Geometry: final body of the model. Coordinates: model frame, mm. Face numbers are marked on the shaded views. A direction names the side the tool comes from. Round coordinates to 2 decimals unless told otherwise and drop trailing zeros. Loops run counter-clockwise (first coordinate to the right, second up) from the corner with the lowest first, then second, coordinate; pieces in that order, holes last. Notation, with made-up numbers: M 65,24 L 85,24 A22 cw 85,47 Z; hole C 7.25,55 d4. An arc over 180 degrees is marked long. Answer as a JSON object with one key per item and string values.
```python
from build123d import *

# Parameters (mm, degrees)
SKETCH1_W           = 60
SKETCH1_H           = 100
SKETCH1_W_2         = 150
SKETCH1_H_2         = 12
BOSS_EXTRUDE1_DEPTH = 30
FILLET1_R           = 10
SKETCH2_W           = 25
SKETCH2_H           = 10
SKETCH2_H_2         = 5
CUT_EXTRUDE1_DEPTH  = 222
FILLET2_R           = 5
SKETCH3_R           = 2
CUT_EXTRUDE2_DEPTH  = 51
SKETCH4_R           = 4
CUT_EXTRUDE3_DEPTH  = 4.5


with BuildPart() as part:
    # Sketch1 → Boss-Extrude1 (new body)
    with BuildSketch(Plane.XY):
        Rectangle(SKETCH1_W, SKETCH1_H)
        with Locations((0, -50)):
            Rectangle(SKETCH1_W_2, SKETCH1_H_2)
    extrude(amount=BOSS_EXTRUDE1_DEPTH)

    # Fillet1
    fillet1_edges = [part.edges().sort_by_distance(p)[0] for p in [
        (-30, -44, 15),
        (30, -44, 15),
    ]]
    fillet(fillet1_edges, radius=FILLET1_R)

    # Sketch2 → Cut-Extrude1 (cut)
    with BuildSketch(Plane(origin=(0, 50, 0), x_dir=(1, 0, 0), z_dir=(0, 1, 0))):
        with Locations((0, -5)):
            Rectangle(SKETCH2_W, SKETCH2_H)
        with Locations((0, -12.5)):
            Rectangle(SKETCH2_W, SKETCH2_H_2)
        Polygon((17.5, -10), (12.5, -10), (12.5, -15), (-12.5, -15), (-12.5, -10), (-17.5, -10), (-17.5, -20), (17.5, -20), align=None)
    extrude(amount=-CUT_EXTRUDE1_DEPTH, mode=Mode.SUBTRACT)

    # Fillet2
    fillet2_edges = [part.edges().sort_by_distance(p)[0] for p in [
        (12.5, 50, 5),
        (-12.5, 50, 5),
        (0, 50, 20),
        (-17.5, 50, 15),
        (17.5, 50, 15),
    ]]
    fillet(fillet2_edges, radius=FILLET2_R)

    # Sketch3 → Cut-Extrude2 (cut)
    with BuildSketch(Plane(origin=(0, -44, 0), x_dir=(1, 0, 0), z_dir=(0, 1, 0))):
        with Locations(Location((-57.5, -15, 0), (0, 0, 270))):
            Circle(SKETCH3_R)
    cut_extrude2 = extrude(amount=-CUT_EXTRUDE2_DEPTH, mode=Mode.SUBTRACT)

    # Sketch4 → Cut-Extrude3 (cut)
    with BuildSketch(Plane(origin=(0, -44, 0), x_dir=(1, 0, 0), z_dir=(0, 1, 0))):
        with Locations(Location((-57.5, -15, 0), (0, 0, 270))):
            Circle(SKETCH4_R)
    cut_extrude3 = extrude(amount=-CUT_EXTRUDE3_DEPTH, mode=Mode.SUBTRACT)

    # Mirror1: Cut-Extrude2, Cut-Extrude3 across plane
    add(cut_extrude2.mirror(Plane(origin=(0, 0, 0), x_dir=(0, 0, 1), z_dir=(1, 0, 0))), mode=Mode.SUBTRACT)
    add(cut_extrude3.mirror(Plane(origin=(0, 0, 0), x_dir=(0, 0, 1), z_dir=(1, 0, 0))), mode=Mode.SUBTRACT)


solid = part.part
```
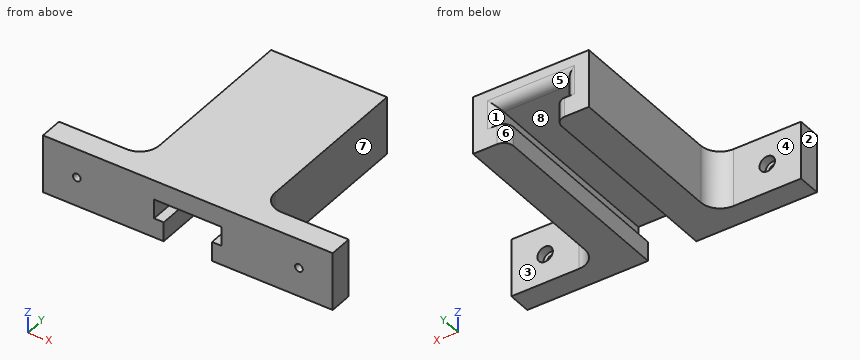
1) First-contact query: pin 1 (9 mm diameter, centred on x = 55.5, z = 15.5, fed in from +Y); pin 2 (11 mm diameter, centred on y = -30, z = 13, fed in from -X); pin 3 (9 mm diameter, centred on x = -57.5, z = 15, fed in from -Y); pin 4 (1 mm diameter, centred on y = 37.5, z = 4, fed in from +X). Flat tips, straight axial feed; report the tip coordinate or a pass-through.
Geometry results:
{"pin 1": "y = -44", "pin 2": "x = -30.11", "pin 3": "y = -56", "pin 4": "x = 30"}
2) Pull-direction query (X, two-part tool) for the marked faces 1, 2 and 3; classes: +X half, -X half, draft (parallel to the pull), parting line (faces both ways), or undercut.
Geometry results:
{"face 1": "undercut", "face 2": "-X half", "face 3": "draft"}
3) Cut plane A-A on x = 57.5. Return the cut outline in (y, z), and give its area (3 significant figures).
Geometry results:
{"outline": "M -56,0 L -44,0 L -44,11 L -48.5,11 L -48.5,13 L -56,13 Z; M -56,17 L -48.5,17 L -48.5,19 L -44,19 L -44,30 L -56,30 Z", "area": "294 mm2"}
4) Cut plane C-C on y = -47. Return the cut outline in (x, z).
Geometry results:
{"outline": "M -75,0 L -12.5,0 L -12.5,10 L -17.5,10 L -17.5,20 L 17.5,20 L 17.5,10 L 12.5,10 L 12.5,0 L 75,0 L 75,30 L -75,30 Z; hole C -57.5,15 d8; hole C 57.5,15 d8"}
5) Cut plane D-D on z = 5.75. Return the cut outline in (x, y).
Geometry results:
{"outline": "M -75,-56 L -12.5,-56 L -12.5,45 A5 ccw -17.5,50 L -30,50 L -30,-34 A10 cw -40,-44 L -75,-44 Z; M 12.5,-56 L 75,-56 L 75,-44 L 40,-44 A10 cw 30,-34 L 30,50 L 17.5,50 A5 ccw 12.5,45 Z"}
6) Set-up query: the marked faces 4, 5, 6, 7 and 8. Return all of +Z, -Z, +X, -X, +Y, -Y with unobstructed straight access to the full face (end or side cutting, diameter ignored); none if empty.
Geometry results:
{"face 4": "+Z, -Z, -X, +Y", "face 5": "+Y", "face 6": "-Z, +Y", "face 7": "+Z, -Z, +X, +Y", "face 8": "+Y, -Y"}
7) Line query: probe 1 along X at (y, z) = (-45.5, 15); probe 2 along X at (y, z) = (-52, 15); probe 3 along Z at (x, y) = (-15.5, 27). Output: solid intervals per line, ascending.
Geometry results:
{"probe 1": "-75 to -61.5, -53.5 to -17.5, 17.5 to 53.5, 61.5 to 75", "probe 2": "-75 to -59.5, -55.5 to -17.5, 17.5 to 55.5, 59.5 to 75", "probe 3": "0 to 10, 20 to 30"}
8) Cut plane B-B on z = 15. Count the separate pieces of the cut face and the enclosed holes in it, and give its area (3 significant figures).
Geometry results:
{"separate pieces": "4", "enclosed holes": "0", "area": "3,630 mm2"}
